Can you work these out from the model? Positions are in its coordinate system, mm. Face numbers are marked on the shaded views. A direction names the side the tool comes from. Give positions to 0.01 mm unless a question says otherwise; leave off trailing zeros. Order: outer loops, then holes, each group sorted by start corner. A loop starts at its lowest first (then second) coordinate and runs counter-clockwise, first axis right, second up.
Item 1: I want a section at C-C, the plane z = 0. Write out the boundary of the cut face in (x, y).
Item 2: I want a section at D-D, the plane x = 7.75. Write out the boundary of the cut face in (y, z) (3 decimals), then the cut area to 3 significant figures.
Item 3: Which directions (+Z, -Z, +X, -X, +Y, -Y) give clear straight access to the entire face, cutting with the end or side of a thin tool? Please do the marked faces 1, 2, 3 and 4.
Item 4: If we mould it in two halves opening along Y, with no side actions, what happens to the marked faces 5, 6 and 7? For each: +Y half, -Y half, draft (parallel to the pull), parting line (faces both ways), or undercut.
Item 5: I want a section at A-A, the plane x = 12.25. Write out the boundary of the cut face in (y, z) (3 decimals), then the cut area to 3 significant figures.
Item 6: If I drill on line 1 along Y through (x, z) = (2.75, 0); line 2 along Z through (x, y) = (14.25, 0); line 3 along X through (y, z) = (11.5, 9.5), over which ranges is the centre line in solid material (lowest first)?
Item 7: I want a section at B-B, the plane y = 0. Write out the boundary of the cut face in (x, z), then the cut area to 3 significant figures.
Item 8: I'm going to push flat-ended pins straight in: pin 1 Ø1.6 at (x, z) = (6, -1) entering from -Y; pin 2 Ø1.6 at (x, z) = (6.5, -4) entering from +Y; pin 3 Ø5.5 at (x, z) = (12.5, 17.5) entering from -Y (3 decimals). Where does each tip first touch, or does it pass through?
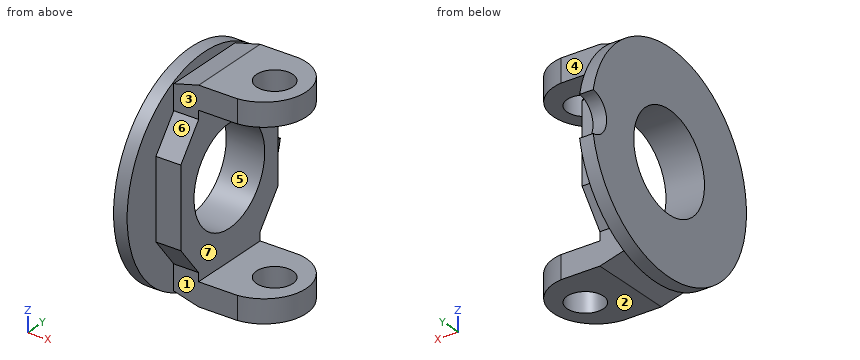
```python
from build123d import *

# Parameters (mm, degrees)
SKETCH1_R           = 10.75
BOSS_EXTRUDE1_DEPTH = 3
SKETCH2_R           = 10.75
BOSS_EXTRUDE2_DEPTH = 5.5
DRAFT1_START        = -9.335
DRAFT1_DEPTH        = 18.67
SKETCH3_W           = 5.13
SKETCH3_H           = 18.67
BOSS_EXTRUDE3_DEPTH = 17
CUT_EXTRUDE1_REACH  = 59.71
CUT_EXTRUDE2_REACH  = 59.71
SKETCH5_R           = 4


# Read off the part's stored shape, not the designer's step: Draft1
with BuildPart() as part:
    # Sketch1 → Boss-Extrude1 (new body)
    with BuildSketch(Plane(origin=(0, 0, 0), x_dir=(0, 0, -1), z_dir=(1, 0, 0))):
        with BuildLine():
            ThreePointArc((-4.479326664, 23.069148936), (0, -23.5), (4.479326664, 23.069148936))
            ThreePointArc((4.479326664, 23.069148936), (0, 19), (-4.479326664, 23.069148936))
        make_face()
        Circle(SKETCH1_R, mode=Mode.SUBTRACT)
    extrude(amount=BOSS_EXTRUDE1_DEPTH)

    # Sketch2 → Boss-Extrude2 (add)
    # profile 1 of 7: a face of its own
    with BuildSketch(Plane(origin=(3, 0, 0), x_dir=(0, 0, -1), z_dir=(1, 0, 0))):
        with BuildLine():
            ThreePointArc((-22.63, 6.33506906), (-22.149027068, 7.853063093), (-21.566357481, 9.335))
            Line((-21.566357481, 9.335), (-22.63, 9.335))
            Line((-22.63, 9.335), (-22.63, 6.33506906))
        make_face()
    # profile 2 of 7: a face of its own
    with BuildSketch(Plane(origin=(3, 0, 0), x_dir=(0, 0, -1), z_dir=(1, 0, 0))):
        with BuildLine():
            Line((-15.63, -9.335), (-15.63, 9.335))
            Line((-15.63, 9.335), (-21.566357481, 9.335))
            ThreePointArc((-21.566357481, 9.335), (-22.149027068, 7.853063093), (-22.63, 6.33506906))
            Line((-22.63, 6.33506906), (-22.63, -6.33506906))
            ThreePointArc((-22.63, -6.33506906), (-22.149027068, -7.853063093), (-21.566357481, -9.335))
            Line((-21.566357481, -9.335), (-15.63, -9.335))
        make_face()
    # profile 3 of 7: a face of its own
    with BuildSketch(Plane(origin=(3, 0, 0), x_dir=(0, 0, -1), z_dir=(1, 0, 0))):
        with BuildLine():
            Line((-22.63, -9.335), (-21.566357481, -9.335))
            ThreePointArc((-21.566357481, -9.335), (-22.149027068, -7.853063093), (-22.63, -6.33506906))
            Line((-22.63, -6.33506906), (-22.63, -9.335))
        make_face()
    # profile 4 of 7: a face of its own
    with BuildSketch(Plane(origin=(3, 0, 0), x_dir=(0, 0, -1), z_dir=(1, 0, 0))):
        Polygon((-8.735, -14.754582548), (8.735, -14.754582548), (15.63, -9.335), (15.63, 9.335), (8.735, 14.754582548), (-8.735, 14.754582548), (-15.63, 9.335), (-15.63, -9.335), align=None)
        Circle(SKETCH2_R, mode=Mode.SUBTRACT)
    # profile 5 of 7: a face of its own
    with BuildSketch(Plane(origin=(3, 0, 0), x_dir=(0, 0, -1), z_dir=(1, 0, 0))):
        with BuildLine():
            Line((21.566357481, 9.335), (15.63, 9.335))
            Line((15.63, 9.335), (15.63, -9.335))
            Line((15.63, -9.335), (21.566357481, -9.335))
            ThreePointArc((21.566357481, -9.335), (22.149027068, -7.853063093), (22.63, -6.33506906))
            Line((22.63, -6.33506906), (22.63, 6.33506906))
            ThreePointArc((22.63, 6.33506906), (22.149027068, 7.853063093), (21.566357481, 9.335))
        make_face()
    # profile 6 of 7: a face of its own
    with BuildSketch(Plane(origin=(3, 0, 0), x_dir=(0, 0, -1), z_dir=(1, 0, 0))):
        with BuildLine():
            ThreePointArc((22.63, -6.33506906), (22.149027068, -7.853063093), (21.566357481, -9.335))
            Line((21.566357481, -9.335), (22.63, -9.335))
            Line((22.63, -9.335), (22.63, -6.33506906))
        make_face()
    # profile 7 of 7: a face of its own
    with BuildSketch(Plane(origin=(3, 0, 0), x_dir=(0, 0, -1), z_dir=(1, 0, 0))):
        with BuildLine():
            Line((22.63, 9.335), (21.566357481, 9.335))
            ThreePointArc((21.566357481, 9.335), (22.149027068, 7.853063093), (22.63, 6.33506906))
            Line((22.63, 6.33506906), (22.63, 9.335))
        make_face()
    extrude(amount=BOSS_EXTRUDE2_DEPTH)

    # Draft1 outline → Draft1 (cut)
    with BuildSketch(Plane(origin=(0, 0, 0), x_dir=(1, 0, 0), z_dir=(0, 1, 0)).offset(DRAFT1_START)):
        Polygon((3, 22.63), (3, 21.156279442), (8.5, 22.63), align=None)
        Polygon((3, -21.156279442), (3, -22.63), (8.5, -22.63), align=None)
    extrude(amount=DRAFT1_DEPTH, mode=Mode.SUBTRACT)

    # Sketch3 → Boss-Extrude3 (add)
    with BuildSketch(Plane(origin=(8.5, 0, 0), x_dir=(0, 0, -1), z_dir=(1, 0, 0))):
        with Locations((-20.065, 0)):
            Rectangle(SKETCH3_W, SKETCH3_H)
        with Locations((20.065, 0)):
            Rectangle(SKETCH3_W, SKETCH3_H)
    extrude(amount=BOSS_EXTRUDE3_DEPTH)

    # Cut-Extrude1: up to this face of the body (flat: up to its plane)
    cut_extrude1_end = Plane(part.part.faces().sort_by_distance((17, 0, -22.63))[0])
    # Sketch4 → Cut-Extrude1 (cut, up to the picked face)
    with BuildSketch(Plane.XY.offset(22.63), mode=Mode.PRIVATE) as cut_extrude1_sk1:
        with BuildLine():
            Line((17.037700932, 12.875), (29.477700932, 12.875))
            Line((29.477700932, 12.875), (29.477700932, -13.095))
            Line((29.477700932, -13.095), (17.037700932, -13.095))
            Line((17.037700932, -13.095), (17.037700932, -9.335))
            ThreePointArc((17.037700932, -9.335), (25.5, 0), (17.037700932, 9.335))
            Line((17.037700932, 9.335), (17.037700932, 12.875))
        make_face()
    cut_extrude1_tool1 = split(extrude(cut_extrude1_sk1.sketch, amount=-CUT_EXTRUDE1_REACH, mode=Mode.PRIVATE), bisect_by=cut_extrude1_end, keep=Keep.BOTH, mode=Mode.PRIVATE)
    add(cut_extrude1_tool1.solids().sort_by(Axis((17.325658, 11.105, 22.63), (0, 0, -1)))[0], mode=Mode.SUBTRACT)

    # Cut-Extrude2: up to this face of the body (flat: up to its plane)
    cut_extrude2_end = Plane(part.part.faces().sort_by_distance((16.149048437, 0, -22.63))[0])
    # Sketch5 → Cut-Extrude2 (cut, up to the picked face)
    with BuildSketch(Plane.XY.offset(22.63), mode=Mode.PRIVATE) as cut_extrude2_sk1:
        with Locations((18.5, 0)):
            Circle(SKETCH5_R)
    cut_extrude2_tool1 = split(extrude(cut_extrude2_sk1.sketch, amount=-CUT_EXTRUDE2_REACH, mode=Mode.PRIVATE), bisect_by=cut_extrude2_end, keep=Keep.BOTH, mode=Mode.PRIVATE)
    add(cut_extrude2_tool1.solids().sort_by(Axis((18.5, 0, 22.63), (0, 0, -1)))[0], mode=Mode.SUBTRACT)


solid = part.part
```
Results list:
1. outline: (0, -23.5) - (3, -23.5) - (3, -14.75) - (8.5, -14.75) - (8.5, -10.75) - (0, -10.75) - close; (0, 10.75) - (8.5, 10.75) - (8.5, 14.75) - (3, 14.75) - (3, 19) - (0, 19) - close
2. outline: (-14.755, -8.735) - (-9.335, -15.63) - (-9.335, -22.429) - (9.335, -22.429) - (9.335, -15.63) - (14.755, -8.735) - (14.755, 8.735) - (9.335, 15.63) - (9.335, 22.429) - (-9.335, 22.429) - (-9.335, 15.63) - (-14.755, 8.735) - close; hole circle Ø21.5 at (0, 0)
2. area: 739 mm2
3. face 1: -Z, +X, -Y
3. face 2: -Z, +X, +Y, -Y
3. face 3: +Z, +X, -Y
3. face 4: +Z, +X, +Y
4. face 5: undercut
4. face 6: -Y half
4. face 7: draft
5. outline: (-9.335, -22.63) - (9.335, -22.63) - (9.335, -17.5) - (-9.335, -17.5) - close; (-9.335, 17.5) - (9.335, 17.5) - (9.335, 22.63) - (-9.335, 22.63) - close
5. area: 192 mm2
6. line 1: y = -23.5 to -10.75, 10.75 to 19
6. line 2: z = -22.63 to -17.5, 17.5 to 22.63
6. line 3: x = 0 to 8.5
7. outline: (0, -23.5) - (3, -23.5) - (3, -21.16) - (8.5, -22.63) - (14.5, -22.63) - (14.5, -17.5) - (8.5, -17.5) - (8.5, -10.75) - (0, -10.75) - close; (0, 10.75) - (8.5, 10.75) - (8.5, 17.5) - (14.5, 17.5) - (14.5, 22.63) - (8.5, 22.63) - (3, 21.16) - (3, 23.5) - (0, 23.5) - close; (22.5, -22.63) - (25.5, -22.63) - (25.5, -17.5) - (22.5, -17.5) - close; (22.5, 17.5) - (25.5, 17.5) - (25.5, 22.63) - (22.5, 22.63) - close
7. area: 291 mm2
8. pin 1: stops at y = -14.75
8. pin 2: stops at y = 14.75
8. pin 3: stops at y = -9.335
